```python
from build123d import *

# Parameters (mm, degrees)
SKETCH1_R           = 15
SKETCH1_R_2         = 2.5
BOSS_EXTRUDE1_DEPTH = 6
FILLET1_R           = 2


with BuildPart() as part:
    # Sketch1 → Boss-Extrude1 (new body)
    with BuildSketch(Plane(origin=(0, 0, 0), x_dir=(0, 0, -1), z_dir=(1, 0, 0))):
        with BuildLine():
            Line((-59.428090416, 18.333333333), (-73.57022604, -21.666666667))
            ThreePointArc((-73.57022604, -21.666666667), (-70.504972651, -44.301961285), (-50.322091296, -54.997925058))
            Line((-50.322091296, -54.997925058), (-7.837413011, -55.545328295))
            Line((-7.837413011, -55.545328295), (-2.444575303, -24.961025846))
            Line((-2.444575303, -24.961025846), (-30.070966116, -14.905841909))
            ThreePointArc((-30.070966116, -14.905841909), (-31.918030616, -12.736095946), (-34, -10.790627288))
            Line((-34, -10.790627288), (-34, 1))
            Line((-34, 1), (-40.649042421, 18.543951518))
            ThreePointArc((-40.649042421, 18.543951518), (-50.11214889, 24.999371112), (-59.428090416, 18.333333333))
        make_face()
        with Locations((-50, -30)):
            Circle(SKETCH1_R, mode=Mode.SUBTRACT)
        with Locations((-50, 15)):
            Circle(SKETCH1_R_2, mode=Mode.SUBTRACT)
        Polygon((-29.84807753, -42.163518223), (-10.15192247, -45.636481777), (-11.193811536, -51.545328295), (-30.889966596, -48.072364741), align=None, mode=Mode.SUBTRACT)
        with BuildLine():
            ThreePointArc((-53.038843109, -2.234135678), (-55.934982936, -4.262034616), (-53.907083998, -7.158174443))
            ThreePointArc((-53.907083998, -7.158174443), (-50, -7.5), (-46.092916002, -7.158174443))
            ThreePointArc((-46.092916002, -7.158174443), (-44.065017064, -4.262034616), (-46.961156891, -2.234135678))
            ThreePointArc((-46.961156891, -2.234135678), (-50, -2.5), (-53.038843109, -2.234135678))
        make_face(mode=Mode.SUBTRACT)
    extrude(amount=BOSS_EXTRUDE1_DEPTH)

    # Fillet1
    fillet1_edges = [part.edges().sort_by_distance(p)[0] for p in [
        (3, -14.905841909, 30.070966116),
        (3, -24.961025846, 2.444575303),
        (3, -55.545328295, 7.837413011),
        (3, 1, 34),
        (3, -10.790627288, 34),
    ]]
    fillet(fillet1_edges, radius=FILLET1_R)


solid = part.part
```
Check sheet for the modelled part. Datum: model origin and axes. Units: mm. A direction names the side the tool comes from. Round coordinates to 2 decimals unless told otherwise and drop trailing zeros. Order: outer loops, then holes, each group sorted by start corner. A loop starts at its lowest first (then second) coordinate and runs counter-clockwise, first axis right, second up. Notation, with made-up numbers: (86, 49.25) -> (120, 49.25) arc R28 ccw to (120, 80.25) -> close; hole circle Ø10 at (5, 80). An arc over 180 degrees is marked (long way). Use CSV: the item, a comma, the result in double quotes.
(1) Draft check along Z on faces 1 (the face through (2.96, -1.39, 66.4)), 2 (the face through (2.958, -29.34, 64.985)), 3 (the face through (3.042, -25.283, 2.964)), 4 (the face through (0, -15, 39)). Enter one of: pulls with the +Z half, pulls with the -Z half, needs draft (parallel to the pull), parting line crosses it, or undercut.
Worked out:
face 1,"pulls with the +Z half"
face 2,"undercut"
face 3,"pulls with the -Z half"
face 4,"needs draft"
(2) Tool access check on faces 5 (the face through (2.958, -49.833, 20.904)), 6 (the face through (3, -5, 34)), 7 (the face through (6, -15, 39)). Record the directions out of +Z, -Z, +X, -X, +Y, -Y that give a thin tool (end or side, any length) a straight path to the whole face; none if there is none.
Worked out:
face 5,"+X, -X"
face 6,"-Z, +X, -X, +Y"
face 7,"+Z, -Z, +X, +Y, -Y"
(3) Depth check by flat-ended pin: pin 1 (1.8 mm diameter, centred on x = 4, y = -6, fed in from -Z). Enter the tip coordinate at first touch or a pass-through.
Worked out:
pin 1,"z = 34"
(4) Cross-section at A-A (x = 3.1). Record the boundary of the cut face in (y, z).
Worked out:
outline,"(-55.52, 9.54) arc R2 ccw to (-53.87, 7.54) -> (-26.61, 2.74) arc R2 ccw to (-24.39, 4.02) -> (-15.1, 29.53) arc R2 cw to (-14.47, 30.41) arc R25 ccw to (-11.37, 33.33) arc R2 cw to (-9.88, 34) -> (0.63, 34) arc R2 ccw to (1.34, 34.13) -> (18.54, 40.65) arc R10 ccw to (18.33, 59.43) -> (-21.67, 73.57) arc R25 ccw to (-55, 50.32) -> close; hole (-51.55, 11.19) -> (-45.64, 10.15) -> (-42.16, 29.85) -> (-48.07, 30.89) -> close; hole circle Ø30 at (-30, 50); hole (-7.16, 46.09) arc R2.5 ccw to (-2.23, 46.96) arc R17.5 cw to (-2.23, 53.04) arc R2.5 ccw to (-7.16, 53.91) arc R22.5 ccw to start; hole circle Ø5 at (15, 50)"
(5) Cross-section at D-D (z = 68). Record the boundary of the cut face in (x, y), and give its area (3 significant figures).
Worked out:
outline,"(0, -47.35) -> (6, -47.35) -> (6, -5.91) -> (0, -5.91) -> close"
area,"249 mm²"
(6) Cross-section at C-C (y = -36). Record the boundary of the cut face in (x, z).
Worked out:
outline,"(0, 4.39) -> (6, 4.39) -> (6, 36.25) -> (0, 36.25) -> close; (0, 63.75) -> (6, 63.75) -> (6, 74.27) -> (0, 74.27) -> close"
(7) Material ranges on line 1 along Y through (x, z) = (2.9, 50); line 2 along Z through (x, y) = (4.05, -27); line 3 along Y through (x, z) = (3.05, 18.5), recorded low to high. Write a range as from..to.
Worked out:
line 1,"-55..-45, -15..-7.5, -2.5..12.5, 17.5..25"
line 2,"2.8..35.3, 64.7..74.82"
line 3,"-55.41..-50.26, -44.16..-19.12"
(8) Cross-section at B-B (z = 18). Record the boundary of the cut face in (x, y).
Worked out:
outline,"(0, -55.41) -> (6, -55.41) -> (6, -50.35) -> (0, -50.35) -> close; (0, -44.25) -> (6, -44.25) -> (6, -19.3) -> (0, -19.3) -> close"
